Could you check a few things on this drawing? It's one solid part, dimensions in mm from its lowest x, y, z. A direction names the side the tool comes from. Give positions to 0.01 mm unless a question says otherwise; leave off trailing zeros. Order: outer loops, then holes, each group sorted by start corner. A loop starts at its lowest first (then second) coordinate and runs counter-clockwise, first axis right, second up.
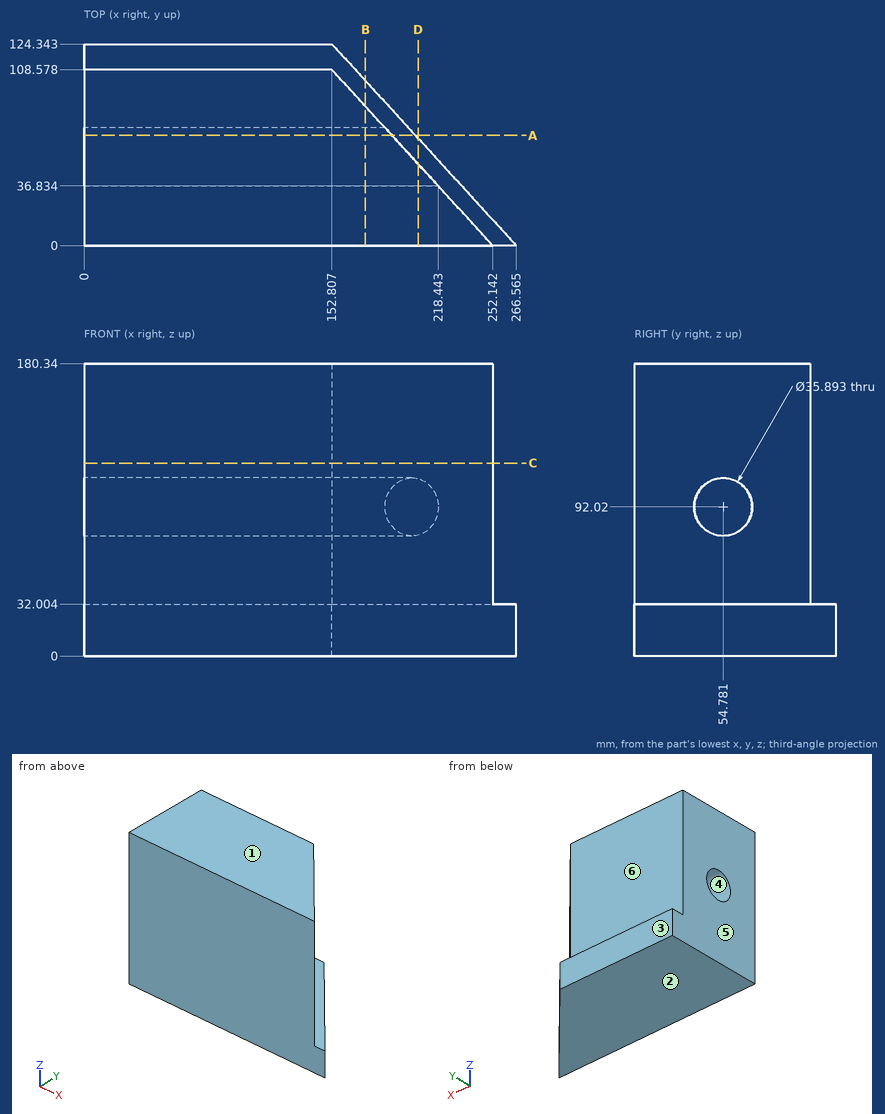
Q1. For the marked faces 5 and 6, which set-ups out of +Z, -Z, +X, -X, +Y, -Y let a thin tool reach every point of the face, with its end or its side?
Filled sheet:
face 5: +Z, -Z, -X, +Y, -Y
face 6: +Z, +X, -X, +Y
Q2. If we section it at B-B on x = 173.5: List the corners of the cut face in (y, z) for me (1 decimal).
Filled sheet:
outline: (0, 0) - (101.7, 0) - (101.7, 32) - (86, 32) - (86, 180.3) - (0, 180.3) - close; hole circle Ø35.9 at (54.8, 92)
Q3. If we section it at A-A on y = 68: List the corners of the cut face in (x, z) for me, plus the area to 3 significant figures.
Filled sheet:
outline: (0, 0) - (204.35, 0) - (204.35, 32) - (189.93, 32) - (189.93, 79.88) - (0, 79.88) - close; (0, 104.16) - (189.93, 104.16) - (189.93, 180.34) - (0, 180.34) - close
area: 30,100 mm2
Q4. If we section it at D-D on x = 206: List the corners of the cut face in (y, z) for me (1 decimal), plus the area to 3 significant figures.
Filled sheet:
outline: (0, 0) - (66.2, 0) - (66.2, 32) - (50.4, 32) - (50.4, 74.6) arc R17.9 cw to (50.4, 109.4) - (50.4, 180.3) - (0, 180.3) - close
area: 9,250 mm2
Q5. Thinking about a two-plate mould opening in Z: for the marked faces 1, 2, 3 and 4, which applies, released by +Z, released by -Z, zero draft, split by the parting line, or undercut?
Filled sheet:
face 1: released by +Z
face 2: released by -Z
face 3: zero draft
face 4: undercut
Q6. I need wall thicknesses on L1, parallel to Y at x = 58.5, z = 93; L2, parallel to Z at x = 176.5, y = 85; L3, parallel to Y at x = 166, z = 12.5. Which ranges of each line are inside material? Lowest first, please.
Filled sheet:
L1: y = 0 to 36.86, 72.7 to 108.58
L2: z = 0 to 32
L3: y = 0 to 109.92
Q7. I'm going to push flat-ended pins straight in: P1, Ø6, axis at x = 41, y = 66.5, coming from the -Z side; P2, Ø6, axis at x = 89.5, z = 94, coming from the +Y side; P3, Ø2, axis at y = 45, z = 71.5, coming from the +X side; P4, Ø3, axis at y = 77, z = 156, coming from the +X side. Where does each tip first touch, or does it pass through?
Filled sheet:
P1: stops at z = 0
P2: stops at y = 108.58
P3: stops at x = 211.89
P4: stops at x = 183.07
Q8. If we section it at C-C on z = 119: List the corners of the cut face in (x, y) for me, plus the area to 3 significant figures.
Filled sheet:
outline: (0, 0) - (252.14, 0) - (152.81, 108.58) - (0, 108.58) - close
area: 22,000 mm2
